from build123d import *

# Parameters (mm, degrees)
F0_R     = 7.5
F0_W     = 52
F0_H     = 52
F1_DEPTH = 10
F2_T     = -2.5
F3_R     = 8


with BuildPart() as f1:
    # F0 (on Top) → F1 (new body)
    with BuildSketch(Plane.XY):
        Polygon((-26, -100), (26, -100), (26, -56), (26, -26), (-26, -26), (-26, -56), align=None)
        with Locations((0, -52.9112443328)):
            Circle(F0_R, mode=Mode.SUBTRACT)
        with BuildLine():
            Line((26, -26), (26, -56))
            ThreePointArc((26, -56), (34.7867965644, -34.7867965644), (56, -26))
            Line((56, -26), (26, -26))
        make_face()
        with BuildLine():
            ThreePointArc((-56, -26), (-34.7867965644, -34.7867965644), (-26, -56))
            Line((-26, -56), (-26, -26))
            Line((-26, -26), (-56, -26))
        make_face()
        Polygon((26, 26), (26, -26), (56, -26), (100, -26), (100, 26), (56, 26), align=None)
        with Locations((59.1130256653, 0)):
            Circle(F0_R, mode=Mode.SUBTRACT)
        Polygon((-56, -26), (-26, -26), (-26, 26), (-56, 26), (-100, 26), (-100, -26), align=None)
        with Locations((-83.977087408, 0)):
            Circle(F0_R, mode=Mode.SUBTRACT)
        Polygon((-26, 26), (26, 26), (26, 56), (26, 100), (-26, 100), (-26, 56), align=None)
        with Locations((0, 52.160911262)):
            Circle(F0_R, mode=Mode.SUBTRACT)
        with BuildLine():
            Line((26, 56), (26, 26))
            Line((26, 26), (56, 26))
            ThreePointArc((56, 26), (34.7867965644, 34.7867965644), (26, 56))
        make_face()
        with BuildLine():
            Line((-56, 26), (-26, 26))
            Line((-26, 26), (-26, 56))
            ThreePointArc((-26, 56), (-34.7867965644, 34.7867965644), (-56, 26))
        make_face()
        Rectangle(F0_W, F0_H)
    extrude(amount=F1_DEPTH)

    # F2
    f2_openings = [f1.faces().sort_by_distance(p)[0] for p in [
        (0.241929, 0.007301, 0),
    ]]
    offset(amount=F2_T, openings=f2_openings)

    # F3
    f3_edges = [f1.edges().sort_by_distance(p)[0] for p in [
        (34.786797, 34.786797, 10),
        (100, 0, 10),
        (78, -26, 10),
        (34.786797, -34.786797, 10),
        (0, 100, 10),
        (-26, 78, 10),
        (-34.786797, -34.786797, 10),
        (-100, 0, 10),
        (0, -100, 10),
    ]]
    fillet(f3_edges, radius=F3_R)


solid = f1.part
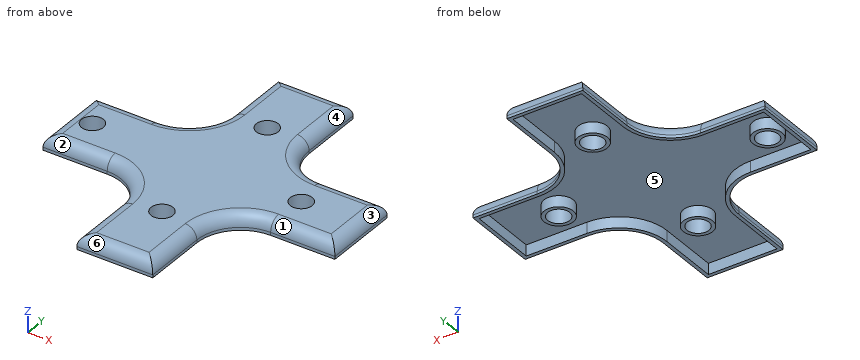
Source: CAD feature listing. Evaluate the final solid. Frame: model axes, mm. Face numbers are marked on the shaded views. A direction names the side the tool comes from. Coordinates: 2 decimals unless noted, no trailing zeros. Loops run counter-clockwise (first coordinate to the right, second up) from the corner with the lowest first, then second, coordinate; pieces in that order, holes last. Notation, with made-up numbers: (-31.75, 48.5) -> (4.25, 48.5) arc R14 cw to (4.25, 75.5) -> close; hole circle Ø10 at (40.25, 24). An arc over 180 degrees is marked (long way). Answer in a Markdown table with one row per item. Add a question column.
Q1. Pull-direction query (Y, two-part tool) for the marked faces 4, 5 and 6; classes: pulls with the +Y half, pulls with the -Y half, needs draft (parallel to the pull), parting line crosses it, or undercut.
Q2. Section A-A on x = 0. Return the cut outline in (y, z).
Q3. Section B-B on y = 0. Return the cut outline in (x, z), and give its area (3 significant figures).
Q4. Ray query, line 1 along X through (y, z) = (-63, 1.5); line 2 along Y through (x, z) = (0, 6.25); line 3 along Y through (x, z) = (0, 4.5). Return the intervals inside material, ascending.
Q5. Section D-D on z = 5.5. Give the number of separate pieces and of enclosed holes in the cut face, and give its area (3 significant figures).
Q6. Contact query for flat-ended pins moving along their axis: pin 1 Ø4 at (x, z) = (75, 4.5) entering from -Y; pin 2 Ø10 at (x, y) = (-45, -12.5) entering from -Z; pin 3 Ø1.6 at (x, z) = (71, 1) entering from +Y. Output: stop coordinate, or through.
Q7. Section C-C on x = 76. Return the cut outline in (y, z), and give its area (3 significant figures).
Q8. Reachability of the marked faces 1, 2 and 3 from +Z, -Z, +X, -X, +Y, -Y: full face, straight path, thin tool, end or side. Return the list, or none.
Computed values:
| question | item | result |
|---|---|---|
| 1 | face 4 | needs draft |
| 1 | face 5 | undercut |
| 1 | face 6 | pulls with the -Y half |
| 2 | outline | (-100, 0) -> (-97.5, 0) -> (-97.5, 7.5) -> (-62.91, 7.5) -> (-62.91, 0) -> (-60.41, 0) -> (-60.41, 10) -> (-92, 10) arc R8 ccw to (-100, 2) -> close; (-45.41, 0) -> (-42.91, 0) -> (-42.91, 7.5) -> (42.16, 7.5) -> (42.16, 0) -> (44.66, 0) -> (44.66, 10) -> (-45.41, 10) -> close; (59.66, 0) -> (62.16, 0) -> (62.16, 7.5) -> (97.5, 7.5) -> (97.5, 0) -> (100, 0) -> (100, 2) arc R8 ccw to (92, 10) -> (59.66, 10) -> close |
| 3 | outline | (-100, 0) -> (-97.5, 0) -> (-97.5, 7.5) -> (-93.98, 7.5) -> (-93.98, 0) -> (-91.48, 0) -> (-91.48, 10) -> (-92, 10) arc R8 ccw to (-100, 2) -> close; (-76.48, 0) -> (-73.98, 0) -> (-73.98, 7.5) -> (49.11, 7.5) -> (49.11, 0) -> (51.61, 0) -> (51.61, 10) -> (-76.48, 10) -> close; (66.61, 0) -> (69.11, 0) -> (69.11, 7.5) -> (97.5, 7.5) -> (97.5, 0) -> (100, 0) -> (100, 2) arc R8 ccw to (92, 10) -> (66.61, 10) -> close |
| 3 | area | 510 mm^2 |
| 4 | line 1 | x = -26 to -23.5, 23.5 to 26 |
| 4 | line 2 | y = -98.78 to -97.5, -62.91 to -60.41, -45.41 to -42.91, 42.16 to 44.66, 59.66 to 62.16, 97.5 to 98.78 |
| 4 | line 3 | y = -99.6 to -97.5, -62.91 to -60.41, -45.41 to -42.91, 42.16 to 44.66, 59.66 to 62.16, 97.5 to 99.6 |
| 5 | separate pieces | 5 |
| 5 | enclosed holes | 5 |
| 5 | area | 1,790 mm^2 |
| 6 | pin 1 | stops at y = -25.98 |
| 6 | pin 2 | stops at z = 7.5 |
| 6 | pin 3 | stops at y = 26 |
| 7 | outline | (-26, 0) -> (-23.5, 0) -> (-23.5, 7.5) -> (23.5, 7.5) -> (23.5, 0) -> (26, 0) -> (26, 2) arc R8 ccw to (18, 10) -> (-18, 10) arc R8 ccw to (-26, 2) -> close |
| 7 | area | 140 mm^2 |
| 8 | face 1 | +Z, +X, -Y |
| 8 | face 2 | +Z, -X, -Y |
| 8 | face 3 | +Z, +X, +Y, -Y |
